Answer from the drawing. Dimensions are ordinates in mm from the lowest x, y and z of the part. A direction names the side the tool comes from. Round coordinates to 2 decimals unless told otherwise and drop trailing zeros. Write each loop counter-clockwise with the first axis right and the second up, starting at its lowest first coordinate (ties: lowest second). Pieces come first, ordered by that corner, then holes. Notation, with made-up numbers: (-17, 41) -> (29, 41) arc R11 cw to (29, 56) -> close; hole circle Ø2 at (-24.5, 64.5). An arc over 180 degrees is marked (long way). Return JSON: item names as keys, results as strings. Group by question number.
(1) Given pin 1 (3 mm diameter, centred on x = 2.5, z = 23, fed in from +Y); pin 2 (14.5 mm diameter, centred on y = 13, z = 13, fed in from -X), each flat-ended and moving along its own axis, determine where each tip first touches the part or whether it passes through.
(2) A cutting plane is placed at D-D on x = 3.5. Give the vertices of the cut face in (y, z).
(3) The mould has two halves that part along Z. Classify the marked faces 1 and 2: released by +Z, released by -Z, zero draft, split by the parting line, or undercut.
(4) A cutting plane is placed at C-C on z = 2.25. Give the vertices of the cut face in (x, y), then the cut area to 3 significant figures.
(5) Straight lines are drawn through the part: line 1 (Y direction, x = 4.85, z = 13); line 2 (Y direction, x = 1.2, z = 13); line 3 (Z direction, x = 1.15, y = 12.25). For each, find the intervals that lie inside material, in ascending order.
(6) For the marked faces 3 and 4, determine the directions among +Z, -Z, +X, -X, +Y, -Y from which every point of the face is accessible in a straight line to the end or side of a thin tool.
(7) A cutting plane is placed at A-A on y = 13. Give the vertices of the cut face in (x, z).
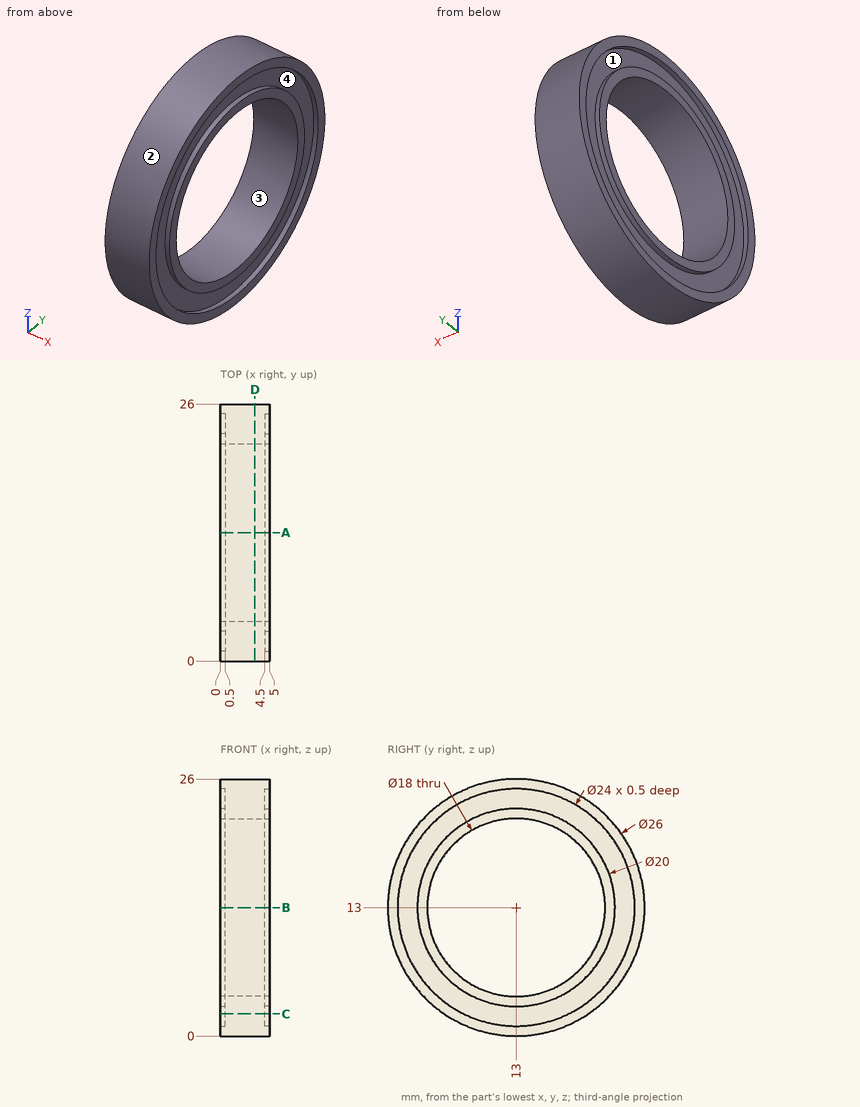
Checks:
{
 "1": {"pin 1": "stops at y = 22.84", "pin 2": "passes through"},
 "2": {"outline": "circle Ø26 at (13, 13); hole circle Ø18 at (13, 13)"},
 "3": {"face 1": "undercut", "face 2": "split by the parting line"},
 "4": {"outline": "(0, 5.69) -> (5, 5.69) -> (5, 7.67) -> (4.5, 7.67) -> (4.5, 18.33) -> (5, 18.33) -> (5, 20.31) -> (0, 20.31) -> (0, 18.33) -> (0.5, 18.33) -> (0.5, 7.67) -> (0, 7.67) -> close", "area": "62.4 mm^2"},
 "5": {"line 1": "y = 0 to 1, 3 to 4, 22 to 23, 25 to 26", "line 2": "y = 0 to 4, 22 to 26", "line 3": "z = 0.02 to 4.03, 21.97 to 25.98"},
 "6": {"face 3": "+X, -X", "face 4": "+X"},
 "7": {"outline": "(0, 0) -> (5, 0) -> (5, 1) -> (4.5, 1) -> (4.5, 3) -> (5, 3) -> (5, 4) -> (0, 4) -> (0, 3) -> (0.5, 3) -> (0.5, 1) -> (0, 1) -> close; (0, 22) -> (5, 22) -> (5, 23) -> (4.5, 23) -> (4.5, 25) -> (5, 25) -> (5, 26) -> (0, 26) -> (0, 25) -> (0.5, 25) -> (0.5, 23) -> (0, 23) -> close"}
}
